CAD build for the part. Positions are in the model's coordinates, mm. A direction names the side the tool comes from. Give positions to 0.01 mm unless a question says otherwise; leave off trailing zeros. Loops run counter-clockwise (first coordinate to the right, second up) from the corner with the lowest first, then second, coordinate; pieces in that order, holes last. Notation, with made-up numbers: (82.5, 34) -> (139.5, 34) arc R14 ccw to (139.5, 41) -> close; hole circle Ø1 at (82, 79.25). An arc over 180 degrees is marked (long way). Use one line per item in the form item = value.
```python
from build123d import *

# Parameters (mm, degrees)
F0_W     = 40.005
F0_H     = 177.8
F1_DEPTH = 3.175
F2_W     = 152.4
F2_H     = 3.175
F3_DEPTH = 3.175
F4_W     = 152.4
F4_H     = 3.175
F5_DEPTH = 3.175


with BuildPart() as f1:
    # F0 (on Top) → F1 (new body)
    with BuildSketch(Plane.XY):
        Rectangle(F0_W, F0_H)
    extrude(amount=F1_DEPTH)

    # F2 (on face) → F3 (join)
    with BuildSketch(Plane(origin=(-20.0025, 0, 0), x_dir=(0, -1, 0), z_dir=(-1, 0, 0))):
        with Locations((0, 1.5875)):
            Rectangle(F2_W, F2_H)
    extrude(amount=F3_DEPTH)

    # F4 (on face) → F5 (join)
    with BuildSketch(Plane.YZ.offset(20.0025)):
        with Locations((0, 1.5875)):
            Rectangle(F4_W, F4_H)
    extrude(amount=F5_DEPTH)


solid = f1.part
```
1. Cut at A-A, the plane z = 0.6. Write the cut outline in (x, y).
Result sheet:
outline = (-23.18, -76.2) -> (-20, -76.2) -> (-20, -88.9) -> (20, -88.9) -> (20, -76.2) -> (23.18, -76.2) -> (23.18, 76.2) -> (20, 76.2) -> (20, 88.9) -> (-20, 88.9) -> (-20, 76.2) -> (-23.18, 76.2) -> close
2. Tool access for faces 1 (the flat face through (-22, -76.2, 2)), 2 (the flat face through (22, -76.2, 2)), 3 (the flat face through (22, 76.2, 2)), 4 (the flat face through (-20.002, 82, 2)): list every direction of +Z, -Z, +X, -X, +Y, -Y with a clear straight run to the whole face (end or side of a thin tool).
Result sheet:
face_1 = +Z, -Z, -X, -Y
face_2 = +Z, -Z, +X, -Y
face_3 = +Z, -Z, +X, +Y
face_4 = +Z, -Z, -X, +Y
3. Drop flat-ended pins along their axis: P1, Ø1, axis at y = -82, z = 2, coming from the -X side; P2, Ø1, axis at y = 82.5, z = 1, coming from the +X side; P3, Ø1.6, axis at x = -21.5, z = 1.5, coming from the +Y side. Give the stop position or say it passes through.
Result sheet:
P1 = -20
P2 = 20
P3 = 76.2
4. Drill centre line: line 1 (X direction, y = 80, z = 1.95). Where is it in solid material? Low to high.
Result sheet:
line_1 = -20 to 20
